Could you check a few things on this model? Use its own coordinates, in mm. A direction names the side the tool comes from. Give positions to 0.01 mm unless a question says otherwise; leave off trailing zeros. Order: outer loops, then holes, each group sorted by start corner. A loop starts at its lowest first (then second) coordinate and runs counter-clockwise, first axis right, second up. Notation, with made-up numbers: M -23,43.5 L 32,43.5 A7 ccw 32,55.5 Z; hole C 12,-24 d5. An arc over 180 degrees is marked long. Use a Markdown table: item, result. Add a question column.
```python
from build123d import *

# Parameters (mm, degrees)
F1_DEPTH = 120
F3_D     = 22
F4_D     = 18
F5_R     = 10
F6_R     = 5


with BuildPart() as f1:
    # F0 (on Front) → F1 (new body)
    with BuildSketch(Plane.XZ):
        Polygon((-200, 10), (-200, 0), (-110, 0), (-110, 105), (110, 105), (110, 0), (200, 0), (200, 10), (120, 10), (120, 115), (-120, 115), (-120, 10), align=None)
    extrude(amount=F1_DEPTH)

    # F3 (through all)
    with Locations(Plane.XY.offset(10)):
        with Locations((160, -50), (-160, -50)):
            Hole(F3_D / 2)

    # F4 (through all)
    with Locations(Plane(origin=(0, 0, 10), x_dir=(1, 0, 0), z_dir=(0, 0, -1))):
        with Locations((0, 60)):
            Hole(F4_D / 2)

    # F5
    f5_edges = [f1.edges().sort_by_distance(p)[0] for p in [
        (-120, -60, 115),
        (120, -60, 115),
        (110, -60, 0),
        (-110, -60, 0),
    ]]
    fillet(f5_edges, radius=F5_R)

    # F6
    f6_edges = [f1.edges().sort_by_distance(p)[0] for p in [
        (-110, -60, 105),
        (110, -60, 105),
        (120, -60, 10),
        (-120, -60, 10),
    ]]
    fillet(f6_edges, radius=F6_R)


solid = f1.part
```
1) Suppose I cut it at D-D on y = -101.5. Please give me the cut outline in (x, z), and give its area (3 significant figures).
2) Suppose I cut it at A-A on z = 84. Please give me the cut outline in (x, y).
3) Suppose I cut it at B-B on x = 160. Please give me the cut outline in (y, z).
4) For faces 5 (the face through (-170, -59, 10)), 6 (the face through (171, -50, 5)), 7 (the face through (112.85, -60.84, 3.01)), 8 (the face through (171, -59, 10)), which set-ups out of +Z, -Z, +X, -X, +Y, -Y let a thin tool reach every point of the face, with its end or its side?
5) Please list where these lines run through material, in increasing order: line 1 (X direction, y = -92, z = 95); line 2 (Y direction, x = -160, z = 3.75); line 3 (Y direction, x = 0, z = 112.5). Write a range as from..to.
6) For pin 1 (20 mm diameter, centred on x = 160, y = -50, fed in from -Z); pin 2 (12 mm diameter, centred on y = -19.5, z = 78, fed in from -X); pin 3 (8 mm diameter, centred on x = 51.5, y = -83.5, fed in from -Z); pin 4 (8 mm diameter, centred on y = -14.5, z = 45, fed in from +X), each with a flat end and sliding along its axis, tell me the tip position at first contact or that it passes through.
7) We'd pull the mould along X, two halves only. Please class faces 1 (the face through (-1, -46, 105)), 2 (the face through (200, -59, 5)), 3 (the face through (-120, -59, 61)), 4 (the face through (151, -59, 0)): pulls with the +X half, pulls with the -X half, needs draft (parallel to the pull), parting line crosses it, or undercut.
8) Suppose I cut it at C-C on y = -43.5. Please give me the cut outline in (x, z), and give its area (3 significant figures).
Values found:
| question | item | result |
|---|---|---|
| 1 | outline | M -200,0 L -120,0 A10 ccw -110,10 L -110,100 A5 cw -105,105 L 105,105 A5 cw 110,100 L 110,10 A10 ccw 120,0 L 200,0 L 200,10 L 125,10 A5 cw 120,15 L 120,105 A10 ccw 110,115 L -110,115 A10 ccw -120,105 L -120,15 A5 cw -125,10 L -200,10 Z |
| 1 | area | 6,040 mm^2 |
| 2 | outline | M -120,-120 L -110,-120 L -110,0 L -120,0 Z; M 110,-120 L 120,-120 L 120,0 L 110,0 Z |
| 3 | outline | M -120,0 L -61,0 L -61,10 L -120,10 Z; M -39,0 L 0,0 L 0,10 L -39,10 Z |
| 4 | face 5 | +Z, -X, +Y, -Y |
| 4 | face 6 | +Z, -Z |
| 4 | face 7 | -Z, +Y, -Y |
| 4 | face 8 | +Z, +X, +Y, -Y |
| 5 | line 1 | x = -120..-110, 110..120 |
| 5 | line 2 | y = -120..-61, -39..0 |
| 5 | line 3 | y = -120..-69, -51..0 |
| 6 | pin 1 | passes through |
| 6 | pin 2 | stops at x = -120 |
| 6 | pin 3 | stops at z = 105 |
| 6 | pin 4 | stops at x = 120 |
| 7 | face 1 | undercut |
| 7 | face 2 | pulls with the +X half |
| 7 | face 3 | pulls with the -X half |
| 7 | face 4 | needs draft |
| 8 | outline | M -200,0 L -168.87,0 L -168.87,10 L -200,10 Z; M -151.13,0 L -120,0 A10 ccw -110,10 L -110,100 A5 cw -105,105 L 105,105 A5 cw 110,100 L 110,10 A10 ccw 120,0 L 151.13,0 L 151.13,10 L 125,10 A5 cw 120,15 L 120,105 A10 ccw 110,115 L -110,115 A10 ccw -120,105 L -120,15 A5 cw -125,10 L -151.13,10 Z; M 168.87,0 L 200,0 L 200,10 L 168.87,10 Z |
| 8 | area | 5,680 mm^2 |
